Work out the finished part from the listing and answer in its coordinate system (mm). A direction names the side the tool comes from. Round coordinates to 2 decimals unless told otherwise and drop trailing zeros. Loops run counter-clockwise (first coordinate to the right, second up) from the corner with the lowest first, then second, coordinate; pieces in that order, holes last.
from build123d import *

# Parameters (mm, degrees)
F0_R     = 44
F0_R_2   = 40
F1_DEPTH = 120
F3_DEPTH = 82
F5_DEPTH = 62.5


with BuildPart() as f1:
    # F0 (on Front) → F1 (new body)
    with BuildSketch(Plane.XZ):
        Circle(F0_R)
        Circle(F0_R_2, mode=Mode.SUBTRACT)
    extrude(amount=F1_DEPTH)

    # F2 (on face) → F3 (cut)
    with BuildSketch(Plane(origin=(0, 0, 0), x_dir=(-1, 0, 0), z_dir=(0, 1, 0))):
        with BuildLine():
            Line((-9.075469, -38.887086), (-10, -42.848571))
            ThreePointArc((-10, -42.848571), (0, -44.049046), (10, -42.848571))
            Line((10, -42.848571), (9.075469, -38.887086))
            ThreePointArc((9.075469, -38.887086), (0, -39.932063), (-9.075469, -38.887086))
        make_face()
        with BuildLine():
            Line((-32.5, 29.66058), (-29.495273, 26.918367))
            ThreePointArc((-29.495273, 26.918367), (0, 39.932063), (29.495273, 26.918367))
            Line((29.495273, 26.918367), (32.5, 29.66058))
            ThreePointArc((32.5, 29.66058), (0, 44.075114), (-32.5, 29.66058))
        make_face()
    extrude(amount=-F3_DEPTH, mode=Mode.SUBTRACT)

    # F4 (on Right) → F5 (cut, symmetric)
    with BuildSketch(Plane.YZ):
        with BuildLine():
            Line((-58.659825, 0), (-98.111279, 0))
            Line((-98.111279, 0), (-98.111279, -23.701457))
            Line((-98.111279, -23.701457), (-35.417102, -23.701457))
            ThreePointArc((-35.417102, -23.701457), (-50.157585, -14.90948), (-58.659825, 0))
        make_face()
    extrude(amount=F5_DEPTH, both=True, mode=Mode.SUBTRACT)


solid = f1.part
Item 1: Section A-A, the plane y = -65.5 is taken. Give the vertices of the cut face in (x, z).
Item 2: Section C-C, the plane z = -12 is taken. Give the vertices of the cut face in (x, y), plus the area to 3 significant figures.
Item 3: Determine the mould class of faces 4 (the face through (0, -82, 41)), 5 (the face through (-9.552, -40.426, -40.928)), 6 (the face through (35, -67, -23.701)) for opening direction Y: pulls with the +Y half, pulls with the -Y half, needs draft (parallel to the pull), parting line crosses it, or undercut.
Item 4: Section D-D, the plane x = 0 is taken. Give the vertices of the cut face in (y, z), plus the area to 3 significant figures.
Item 5: Section B-B, the plane y = -85.5 is taken. Give the vertices of the cut face in (x, z), plus the area to 3 significant figures.
Item 6: Straight lines are drawn through the part: line 1 (Z direction, x = 0, y = -86); line 2 (X direction, y = -101, z = -24.5). For each, find the intervals that lie inside material, in ascending order.
Item 7: Each of these flat-tipped pins is pushed along its axis until it touches: P1, Ø9.5, axis at x = -41, z = -10, coming from the +Y side; P2, Ø8, axis at y = -104.5, z = 13, coming from the -X side; P3, Ø13.5, axis at x = -7.5, z = 39.5, coming from the +Y side; P4, Ø2, axis at x = -21, y = -55, coming from the +Z side. Where does it stop, or does it pass through?
Item 8: For faces 1 (the face through (-40, -98.111, -12)), 2 (the face through (42, -78, 0)), 3 (the face through (31.04, -40.43, 28.33)), determine the directions among +Z, -Z, +X, -X, +Y, -Y from which every point of the face is accessible in a straight line to the end or side of a thin tool.
Answer below:
1. outline: (-44, 0) - (-40, 0) arc R40 cw to (-29.55, 26.96) - (-32.5, 29.66) arc R44 ccw to start; (-37.07, -23.7) arc R44 ccw to (-10, -42.85) - (-9.09, -38.95) arc R40 cw to (-32.22, -23.7) - close; (9.09, -38.95) - (10, -42.85) arc R44 ccw to (37.07, -23.7) - (32.22, -23.7) arc R40 cw to start; (29.55, 26.96) arc R40 cw to (40, 0) - (44, 0) arc R44 ccw to (32.5, 29.66) - close
2. outline: (-42.33, -120) - (-38.16, -120) - (-38.16, -98.11) - (-42.33, -98.11) - close; (-42.33, -52.7) - (-38.16, -52.7) - (-38.16, 0) - (-42.33, 0) - close; (38.16, -120) - (42.33, -120) - (42.33, -98.11) - (38.16, -98.11) - close; (38.16, -52.7) - (42.33, -52.7) - (42.33, 0) - (38.16, 0) - close
2. area: 623 mm2
3. face 4: pulls with the +Y half
3. face 5: needs draft
3. face 6: undercut
4. outline: (-120, -44) - (-82, -44) - (-82, -40) - (-120, -40) - close; (-120, 40) - (-82, 40) - (-82, 44) - (-120, 44) - close
4. area: 304 mm2
5. outline: (-44, 0) - (-40, 0) arc R40 cw to (40, 0) - (44, 0) arc R44 ccw to start; (-37.07, -23.7) arc R44 ccw to (37.07, -23.7) - (32.22, -23.7) arc R40 cw to (-32.22, -23.7) - close
5. area: 854 mm2
6. line 1: z = -44 to -40, 40 to 44
6. line 2: x = -36.55 to -31.62, 31.62 to 36.55
7. P1: stops at y = 0
7. P2: stops at x = -43.07
7. P3: stops at y = -82
7. P4: stops at z = -33.41
8. face 1: +X, -X
8. face 2: -Z, +X, -X
8. face 3: +Z, +Y
